Work out the finished part from the listing and answer in its coordinate system (mm). A direction names the side the tool comes from. Round coordinates to 2 decimals unless told otherwise and drop trailing zeros. Loops run counter-clockwise (first coordinate to the right, second up) from the corner with the lowest first, then second, coordinate; pieces in that order, holes last. Notation, with made-up numbers: M -20,-30 L 2,-30 A14 cw 2,-20 Z; hole C -17,-11.75 d2. An arc over 180 degrees is marked long. One line per item, written item: value.
```python
from build123d import *

# Parameters (mm, degrees)
BOSS_EXTRUDE1_DEPTH  = 0.79375
M2_CLEARANCE_HOLE1_D = 2.6
FILLET1_R            = 4.5
M2_CLEARANCE_HOLE3_D = 2.6
FILLET2_R            = 9
M2_CLEARANCE_HOLE2_D = 2.4
FILLET3_R            = 6
FILLET4_R            = 20
FILLET5_R            = 16
CUT_EXTRUDE2_REACH   = 165.486
CUT_EXTRUDE4_DEPTH   = 164.485535006
M2_CLEARANCE_HOLE4_D = 2.4
SKETCH17_R           = 1.575
CUT_EXTRUDE6_DEPTH   = 164.485535006


with BuildPart() as part:
    # Sketch1 → Boss-Extrude1 (new, symmetric)
    with BuildSketch(Plane(origin=(0, 0, 0), x_dir=(1, 0, 0), z_dir=(0, 1, 0))):
        Polygon((-65, -150), (65, -150), (65, -124), (36, -113.444863206), (36, -25), (63.5, -25), (63.5, 0), (-63.5, 0), (-63.5, -25), (-36, -25), (-36, -113.444863206), (-65, -124), align=None)
    extrude(amount=BOSS_EXTRUDE1_DEPTH, both=True)

    # M2 Clearance Hole1 (through all)
    with Locations(Plane(origin=(0, 0.79375, 0), x_dir=(1, 0, 0), z_dir=(0, 1, 0))):
        with Locations((-60.5, -145.5), (60.5, -145.5), (-60.5, -127.5), (60.5, -127.5), (-28, -127.5), (-28, -145.5), (28, -127.5), (28, -145.5)):
            Hole(M2_CLEARANCE_HOLE1_D / 2)

    # Fillet1
    fillet1_edges = [part.edges().sort_by_distance(p)[0] for p in [
        (65, 0, 150),
        (-65, 0, 150),
    ]]
    fillet(fillet1_edges, radius=FILLET1_R)

    # M2 Clearance Hole3 (through all)
    with Locations(Plane(origin=(0, 0.79375, 0), x_dir=(1, 0, 0), z_dir=(0, 1, 0))):
        with Locations((24.13, -94.7), (8.89, -145.5), (-24.13, -93.43)):
            Hole(M2_CLEARANCE_HOLE3_D / 2)

    # Fillet2
    fillet2_edges = [part.edges().sort_by_distance(p)[0] for p in [
        (-63.5, 0, 0),
        (63.5, 0, 0),
    ]]
    fillet(fillet2_edges, radius=FILLET2_R)

    # M2 Clearance Hole2 (through all)
    with Locations(Plane(origin=(0, 0.79375, 0), x_dir=(1, 0, 0), z_dir=(0, 1, 0))):
        with Locations((-58.42, -13.57), (58.42, -13.57)):
            Hole(M2_CLEARANCE_HOLE2_D / 2)

    # Fillet3
    fillet3_edges = [part.edges().sort_by_distance(p)[0] for p in [
        (-65, 0, 124),
        (65, 0, 124),
    ]]
    fillet(fillet3_edges, radius=FILLET3_R)

    # Fillet4
    fillet4_edges = [part.edges().sort_by_distance(p)[0] for p in [
        (-36, 0, 113.444863206),
        (36, 0, 113.444863206),
    ]]
    fillet(fillet4_edges, radius=FILLET4_R)

    # Fillet5
    fillet5_edges = [part.edges().sort_by_distance(p)[0] for p in [
        (-36, 0, 25),
        (36, 0, 25),
    ]]
    fillet(fillet5_edges, radius=FILLET5_R)

    # Sketch9 → Cut-Extrude2 (cut, up to next)
    with BuildSketch(Plane(origin=(0, 0.79375, 0), x_dir=(1, 0, 0), z_dir=(0, 1, 0)), mode=Mode.PRIVATE) as cut_extrude2_sk1:
        with BuildLine():
            Line((-13, -46), (13, -46))
            ThreePointArc((13, -46), (17, -50), (13, -54))
            Line((13, -54), (-13, -54))
            ThreePointArc((-13, -54), (-17, -50), (-13, -46))
        make_face()
    cut_extrude2_tool1 = extrude(cut_extrude2_sk1.sketch, amount=-CUT_EXTRUDE2_REACH, mode=Mode.PRIVATE) & part.part
    add(cut_extrude2_tool1.solids().sort_by_distance((0, 0.79375, 50))[0], mode=Mode.SUBTRACT)

    # Sketch13 → Cut-Extrude4 (cut, through all)
    with BuildSketch(Plane(origin=(0, 0.79375, 0), x_dir=(1, 0, 0), z_dir=(0, 1, 0))):
        with BuildLine():
            Line((-35, -131), (-35, -142))
            ThreePointArc((-35, -142), (-35.878679656, -144.121320344), (-38, -145))
            Line((-38, -145), (-45.5, -145))
            ThreePointArc((-45.5, -145), (-47.621320344, -144.121320344), (-48.5, -142))
            Line((-48.5, -142), (-48.5, -131))
            ThreePointArc((-48.5, -131), (-47.621320344, -128.878679656), (-45.5, -128))
            Line((-45.5, -128), (-38, -128))
            ThreePointArc((-38, -128), (-35.878679656, -128.878679656), (-35, -131))
        make_face()
        with BuildLine():
            Line((35, -131), (35, -142))
            ThreePointArc((35, -142), (35.878679656, -144.121320344), (38, -145))
            Line((38, -145), (45.5, -145))
            ThreePointArc((45.5, -145), (47.621320344, -144.121320344), (48.5, -142))
            Line((48.5, -142), (48.5, -131))
            ThreePointArc((48.5, -131), (47.621320344, -128.878679656), (45.5, -128))
            Line((45.5, -128), (38, -128))
            ThreePointArc((38, -128), (35.878679656, -128.878679656), (35, -131))
        make_face()
    extrude(amount=-CUT_EXTRUDE4_DEPTH, mode=Mode.SUBTRACT)

    # M2 Clearance Hole4 (through all)
    with Locations(Plane(origin=(0, 0.79375, 0), x_dir=(1, 0, 0), z_dir=(0, 1, 0))):
        with Locations((-7.366, -64), (7.366, -64)):
            Hole(M2_CLEARANCE_HOLE4_D / 2)

    # Sketch17 → Cut-Extrude6 (cut, through all)
    with BuildSketch(Plane(origin=(0, 0.79375, 0), x_dir=(1, 0, 0), z_dir=(0, 1, 0))):
        with Locations(Location((7.8, -18.5, 0), (0, 0, 270))):
            Circle(SKETCH17_R)
        with Locations(Location((-10.2, -18.5, 0), (0, 0, 270))):
            Circle(SKETCH17_R)
        with Locations(Location((36.35, -10.6, 0), (0, 0, 270))):
            Circle(SKETCH17_R)
        with Locations(Location((13.65, -10.6, 0), (0, 0, 270))):
            Circle(SKETCH17_R)
        with Locations(Location((-13.65, -10.6, 0), (0, 0, 270))):
            Circle(SKETCH17_R)
        with Locations(Location((-36.35, -10.6, 0), (0, 0, 270))):
            Circle(SKETCH17_R)
    extrude(amount=-CUT_EXTRUDE6_DEPTH, mode=Mode.SUBTRACT)


solid = part.part
```
1) For faces 5 (the face through (-17, 0, 50)), 6 (the face through (55.19, 0.01, 120.43)), 7 (the face through (-63.885, -0.011, 124.718)), determine the directions among +Z, -Z, +X, -X, +Y, -Y from which every point of the face is accessible in a straight line to the end or side of a thin tool.
Check values:
face 5: +Y, -Y
face 6: +X, +Y, -Y
face 7: -X, +Y, -Y
2) Find section C-C (z = 28.5). Give the vertices of the cut face in (x, y), then the cut area to 3 significant figures.
Check values:
outline: M -42.01,-0.79 L 42.01,-0.79 L 42.01,0.79 L -42.01,0.79 Z
area: 133 mm2
3) Find the intervals of material crossed by probe 1 along X at (y, z) = (-0.65, 134.5); probe 2 along Z at (x, y) = (-58.5, -0.6); probe 3 along Z at (x, y) = (-10, -0.4), in increasing order. Write a range as from..to.
Check values:
probe 1: -65..-48.5, -35..35, 48.5..65
probe 2: 0.94..12.37, 14.77..25, 121.63..150
probe 3: 0..16.94, 20.06..46, 54..150
4) Find section A-A (z = 50). Give the vertices of the cut face in (x, y).
Check values:
outline: M -36,-0.79 L -17,-0.79 L -17,0.79 L -36,0.79 Z; M 17,-0.79 L 36,-0.79 L 36,0.79 L 17,0.79 Z
5) Find section B-B (y = 0.4). Give the number of separate pieces and of enclosed holes in the cut face, then the cut area to 3 significant figures.
Check values:
separate pieces: 1
enclosed holes: 24
area: 13,300 mm2
6) The mould has two halves that part along X. Classify faces 1 (the face through (37.91, 0.01, 10.39)), 2 (the face through (40.811, 0.011, 29.563)), 3 (the face through (-39.716, -0.011, 111.052)), 4 (the face through (47.6, 0.01, 144.14)): +X half, -X half, draft (parallel to the pull), parting line (faces both ways), or undercut.
Check values:
face 1: undercut
face 2: +X half
face 3: -X half
face 4: undercut
7) Each of these flat-tipped pins is pushed along its axis until it touches: pin 1 (0.8 mm diameter, centred on y = -0.5, z = 72.5, fed in from +X); pin 2 (3.5 mm diameter, centred on x = -60.5, z = 145.5, fed in from +Y); pin 3 (2 mm diameter, centred on x = -28, z = 127.5, fed in from -Y). Where does it stop, or does it pass through?
Check values:
pin 1: x = 36
pin 2: y = 0.79
pin 3: through
